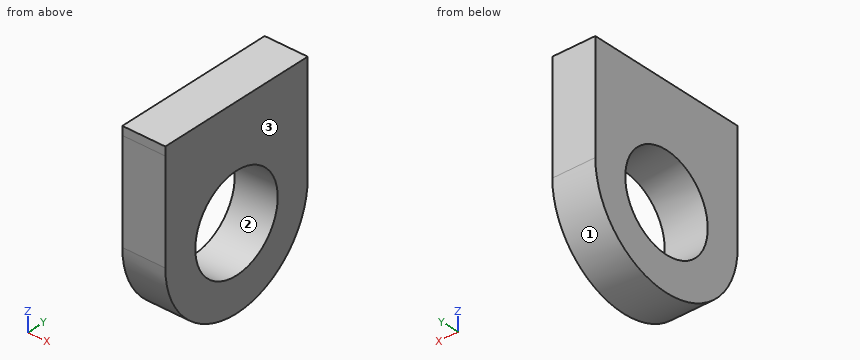
from build123d import *

# Parameters (mm, degrees)
BOSS_EXTRUDE1_DEPTH = 10
SKETCH2_R           = 11
CUT_EXTRUDE1_DEPTH  = 10
BOSS_EXTRUDE2_START = -37.960973
SKETCH3_W           = 10
SKETCH3_H           = 2
BOSS_EXTRUDE2_DEPTH = 37.960973


with BuildPart() as part:
    # Sketch1 → Boss-Extrude1 (new body)
    with BuildSketch(Plane(origin=(0, 0, 0), x_dir=(0, 0, -1), z_dir=(1, 0, 0))):
        with BuildLine():
            Line((-23.5, 18.980486252), (0, 18.980486252))
            ThreePointArc((0, 18.980486252), (18.980486252, 0), (0, -18.980486252))
            Line((0, -18.980486252), (-23.5, -18.980486252))
            Line((-23.5, -18.980486252), (-23.5, 18.980486252))
        make_face()
    extrude(amount=BOSS_EXTRUDE1_DEPTH)

    # Sketch2 → Cut-Extrude1 (cut)
    with BuildSketch(Plane.ZY):
        Circle(SKETCH2_R)
    extrude(amount=-CUT_EXTRUDE1_DEPTH, mode=Mode.SUBTRACT)

    # Sketch3 → Boss-Extrude2 (add)
    with BuildSketch(Plane(origin=(0, 18.980486252, 0), x_dir=(1, 0, 0), z_dir=(0, 1, 0)).offset(BOSS_EXTRUDE2_START)):
        with Locations((5, -24.5)):
            Rectangle(SKETCH3_W, SKETCH3_H)
    extrude(amount=BOSS_EXTRUDE2_DEPTH)


solid = part.part
Work out the finished part from the listing and answer in its coordinate system (mm). Face numbers are marked on the shaded views. Give positions to 0.01 mm unless a question says otherwise; leave off trailing zeros. Order: outer loops, then holes, each group sorted by start corner. A loop starts at its lowest first (then second) coordinate and runs counter-clockwise, first axis right, second up. Notation, with made-up numbers: (34.5, -12) -> (50.5, -12) arc R20 cw to (50.5, -8) -> close; hole circle Ø10 at (8.25, -35.75). An arc over 180 degrees is marked (long way). Answer as a JSON object with one key per item and string values. Group by question number.
1. Section D-D on y = 11.5 is taken. Determine the outline of the cut face in (x, z).
2. Section B-B on x = 5.5 is taken. Determine the outline of the cut face in (y, z).
3. Section C-C on z = 7.5 is taken. Determine the outline of the cut face in (x, y), plus the area to 3 significant figures.
4. Consider line 1 along Y through (x, z) = (6.5, 0); line 2 along Y through (x, z) = (1, -3); line 3 along Z through (x, y) = (3.25, -2). Determine where each line is inside the solid, lowest interval first. Write a range as [from, to].
5. The mould has two halves that part along Y. Classify the marked faces 1, 2 and 3: released by +Y, released by -Y, zero draft, split by the parting line, or undercut.
6. Flat-ended cylindrical pins translate along their axes: pin 1 Ø4 at (x, z) = (4.5, -3) entering from -Y; pin 2 Ø1 at (x, y) = (6, -7) entering from -Z; pin 3 Ø1 at (x, y) = (5.5, 4.5) entering from -Z. Find the tip coordinate at first contact, or state that the pin passes through.
7. Section A-A on y = 0 is taken. Determine the outline of the cut face in (x, z).
Result sheet:
{
 "1": {"outline": "(0, -15.1) -> (10, -15.1) -> (10, 25.5) -> (0, 25.5) -> close"},
 "2": {"outline": "(-18.98, 0) arc R18.98 ccw to (18.98, 0) -> (18.98, 25.5) -> (-18.98, 25.5) -> close; hole circle Ø22 at (0, 0)"},
 "3": {"outline": "(0, -18.98) -> (10, -18.98) -> (10, -8.05) -> (0, -8.05) -> close; (0, 8.05) -> (10, 8.05) -> (10, 18.98) -> (0, 18.98) -> close", "area": "219 mm^2"},
 "4": {"line 1": "y = [-18.98, -11], [11, 18.98]", "line 2": "y = [-18.74, -10.58], [10.58, 18.74]", "line 3": "z = [-18.87, -10.82], [10.82, 25.5]"},
 "5": {"face 1": "split by the parting line", "face 2": "undercut", "face 3": "zero draft"},
 "6": {"pin 1": "stops at y = -18.95", "pin 2": "stops at z = -17.83", "pin 3": "stops at z = -18.55"},
 "7": {"outline": "(0, -18.98) -> (10, -18.98) -> (10, -11) -> (0, -11) -> close; (0, 11) -> (10, 11) -> (10, 25.5) -> (0, 25.5) -> close"}
}
